Check sheet for the modelled part. Datum: model origin and axes. Units: mm. Face numbers are marked on the shaded views. A direction names the side the tool comes from. Round coordinates to 2 decimals unless told otherwise and drop trailing zeros. Write each loop counter-clockwise with the first axis right and the second up, starting at its lowest first coordinate (ties: lowest second). Pieces come first, ordered by that corner, then holes. Notation, with made-up numbers: (-21, -18.75) -> (18, -18.75) arc R21 cw to (18, 11.25) -> close; hole circle Ø2 at (-10.75, 49). An arc over 180 degrees is marked (long way). One line per item, written item: value.
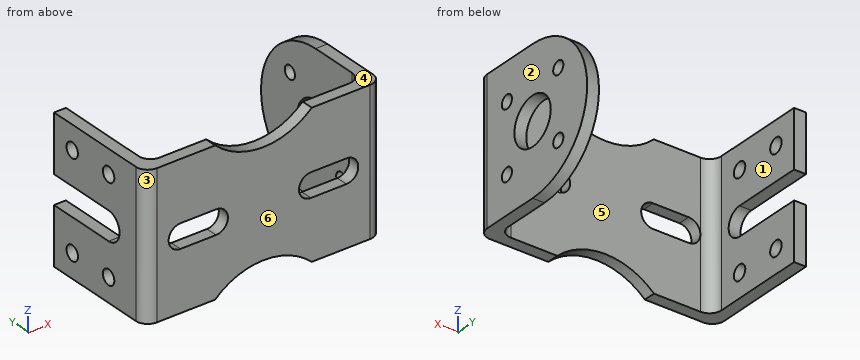
from build123d import *

# Parameters (mm, degrees)
SALIENTE_EXTRUIR1_DEPTH = 5
CROQUIS2_R              = 10.000000000000002
CROQUIS2_R_2            = 2.7999999999999976
CROQUIS2_R_3            = 2.800000000000002
SALIENTE_EXTRUIR2_DEPTH = 5
CROQUIS3_R              = 3.149999999999999
CROQUIS3_R_2            = 3.1499999999999972
SALIENTE_EXTRUIR3_DEPTH = 5
REDONDEO1_R             = 5
REDONDEO2_R             = 5
REDONDEO3_R             = 5
REDONDEO4_R             = 5


with BuildPart() as part:
    # Croquis1 → Saliente-Extruir1 (new body)
    with BuildSketch(Plane(origin=(0, 0, 0), x_dir=(1, 0, 0), z_dir=(0, 1, 0))):
        with BuildLine():
            Line((-46.42082429501085, 21.041214750542295), (-16.81690234938199, 21.041214750542295))
            ThreePointArc((-16.81690234938199, 21.041214750542295), (3.579175704989149, 13.041214750542295), (23.975253759360285, 21.041214750542295))
            Line((23.975253759360285, 21.041214750542295), (53.57917570498915, 21.041214750542295))
            Line((53.57917570498915, 21.041214750542295), (53.57917570498915, -38.9587852494577))
            Line((53.57917570498915, -38.9587852494577), (23.975253759360285, -38.9587852494577))
            ThreePointArc((23.975253759360285, -38.9587852494577), (3.579175704989149, -30.958785249457698), (-16.81690234938199, -38.9587852494577))
            Line((-16.81690234938199, -38.9587852494577), (-46.420824295010846, -38.9587852494577))
            Line((-46.420824295010846, -38.9587852494577), (-46.42082429501085, 21.041214750542295))
        make_face()
        with BuildLine():
            Line((-16.42082429501085, -3.958785249457704), (-31.42082429501085, -3.9587852494577107))
            ThreePointArc((-31.42082429501085, -3.9587852494577107), (-36.420824295010846, -8.958785249457705), (-31.42082429501085, -13.9587852494577))
            Line((-31.42082429501085, -13.9587852494577), (-16.42082429501085, -13.958785249457705))
            ThreePointArc((-16.42082429501085, -13.958785249457705), (-11.42082429501085, -8.958785249457705), (-16.42082429501085, -3.958785249457704))
        make_face(mode=Mode.SUBTRACT)
        with BuildLine():
            Line((23.579175704989144, -13.958785249457705), (38.57917570498914, -13.9587852494577))
            ThreePointArc((38.57917570498914, -13.9587852494577), (43.57917570498913, -8.958785249457705), (38.57917570498914, -3.9587852494577107))
            Line((38.57917570498914, -3.9587852494577107), (23.579175704989144, -3.958785249457704))
            ThreePointArc((23.579175704989144, -3.958785249457704), (18.579175704989144, -8.958785249457705), (23.579175704989144, -13.958785249457705))
        make_face(mode=Mode.SUBTRACT)
    extrude(amount=SALIENTE_EXTRUIR1_DEPTH)

    # Croquis2 → Saliente-Extruir2 (add)
    with BuildSketch(Plane(origin=(53.57917570498915, 0, 0), x_dir=(0, 0, -1), z_dir=(1, 0, 0))):
        with BuildLine():
            Line((-38.9587852494577, 0), (21.0412147505423, 0))
            Line((21.0412147505423, 0), (21.0412147505423, 30))
            ThreePointArc((21.0412147505423, 30), (-8.9587852494577, 60), (-38.9587852494577, 30))
            Line((-38.9587852494577, 30), (-38.9587852494577, 0))
        make_face()
        with Locations((-8.958785249457701, 30)):
            Circle(CROQUIS2_R, mode=Mode.SUBTRACT)
        with Locations((-23.10092087318865, 44.14213562373096)):
            Circle(CROQUIS2_R_2, mode=Mode.SUBTRACT)
        with Locations((-23.100920873188652, 15.85786437626905)):
            Circle(CROQUIS2_R_3, mode=Mode.SUBTRACT)
        with Locations(Location((5.183350374273251, 15.85786437626905, 0), (0, 0, 180))):
            Circle(CROQUIS2_R_3, mode=Mode.SUBTRACT)
        with Locations(Location((5.183350374273248, 44.14213562373096, 0), (0, 0, 180))):
            Circle(CROQUIS2_R_2, mode=Mode.SUBTRACT)
    extrude(amount=-SALIENTE_EXTRUIR2_DEPTH)

    # Croquis3 → Saliente-Extruir3 (add)
    with BuildSketch(Plane.ZY.offset(46.42082429501085)):
        with BuildLine():
            Line((-21.041214750542302, 0), (38.9587852494577, 0))
            Line((38.9587852494577, 0), (38.9587852494577, 50))
            Line((38.9587852494577, 50), (14.958785249457705, 50))
            Line((14.958785249457705, 50), (14.958785249457707, 20.000000000000004))
            ThreePointArc((14.958785249457707, 20.000000000000004), (8.958785249457703, 14.000000000000004), (2.958785249457704, 20.000000000000004))
            Line((2.958785249457704, 20.000000000000004), (2.9587852494577036, 50))
            Line((2.9587852494577036, 50), (-21.041214750542302, 50))
            Line((-21.041214750542302, 50), (-21.041214750542302, 0))
        make_face()
        with Locations((-11.041214750542295, 19.999999999999996)):
            Circle(CROQUIS3_R, mode=Mode.SUBTRACT)
        with Locations((-11.041214750542295, 39.99999999999999)):
            Circle(CROQUIS3_R, mode=Mode.SUBTRACT)
        with Locations(Location((28.958785249457705, 20.000000000000004, 0), (0, 0, 180))):
            Circle(CROQUIS3_R, mode=Mode.SUBTRACT)
        with Locations(Location((28.958785249457698, 40.00000000000001, 0), (0, 0, 180))):
            Circle(CROQUIS3_R_2, mode=Mode.SUBTRACT)
    extrude(amount=-SALIENTE_EXTRUIR3_DEPTH)

    # Redondeo1
    redondeo1_edges = [part.edges().sort_by_distance(p)[0] for p in [
        (-41.42082429501085, 5, 8.9587852494577),
    ]]
    fillet(redondeo1_edges, radius=REDONDEO1_R)

    # Redondeo2
    redondeo2_edges = [part.edges().sort_by_distance(p)[0] for p in [
        (48.57917570498915, 5, 8.958785249457703),
    ]]
    fillet(redondeo2_edges, radius=REDONDEO2_R)

    # Redondeo3
    redondeo3_edges = [part.edges().sort_by_distance(p)[0] for p in [
        (53.57917570498915, 0, 8.958785249457701),
    ]]
    fillet(redondeo3_edges, radius=REDONDEO3_R)

    # Redondeo4
    redondeo4_edges = [part.edges().sort_by_distance(p)[0] for p in [
        (-46.420824295010846, 0, 8.958785249457701),
    ]]
    fillet(redondeo4_edges, radius=REDONDEO4_R)


solid = part.part
Item 1: Tool access check on the marked faces 5 and 6. Record the directions out of +Z, -Z, +X, -X, +Y, -Y that give a thin tool (end or side, any length) a straight path to the whole face; none if there is none.
Result set:
face 5: +Z, -Z, +Y
face 6: +Z, -Z, +X, -X, -Y
Item 2: Sectioned sample at A-A (x = 37.5). Enter the section's corners in (y, z).
Result set:
outline: (0, -21.04) -> (5, -21.04) -> (5, 3.96) -> (0, 3.96) -> close; (0, 13.96) -> (5, 13.96) -> (5, 38.96) -> (0, 38.96) -> close
Item 3: Release check for a two-part mould opening along X. For the marked faces 1, 2, 3 and 4 record: pulls with the +X half, pulls with the -X half, needs draft (parallel to the pull), parting line crosses it, or undercut.
Result set:
face 1: undercut
face 2: pulls with the +X half
face 3: pulls with the -X half
face 4: needs draft
Item 4: Sectioned sample at B-B (z = -16.5). Enter the section's corners in (x, y), then the cut area to 3 significant figures.
Result set:
outline: (-46.42, 5) arc R5 ccw to (-41.42, 0) -> (-10.41, 0) -> (-10.41, 5) -> (-36.42, 5) arc R5 cw to (-41.42, 10) -> (-41.42, 50) -> (-46.42, 50) -> close; (17.56, 0) -> (48.58, 0) arc R5 ccw to (53.58, 5) -> (53.58, 45.87) -> (48.58, 45.87) -> (48.58, 10) arc R5 cw to (43.58, 5) -> (17.56, 5) -> close
area: 790 mm^2
Item 5: Sectioned sample at C-C (z = 27). Enter the section's corners in (x, y).
Result set:
outline: (-46.42, 5) arc R5 ccw to (-41.42, 0) -> (48.58, 0) arc R5 ccw to (53.58, 5) -> (53.58, 53.97) -> (48.58, 53.97) -> (48.58, 10) arc R5 cw to (43.58, 5) -> (-36.42, 5) arc R5 cw to (-41.42, 10) -> (-41.42, 17.53) -> (-46.42, 17.53) -> close; (-46.42, 22.47) -> (-41.42, 22.47) -> (-41.42, 37.53) -> (-46.42, 37.53) -> close; (-46.42, 42.47) -> (-41.42, 42.47) -> (-41.42, 50) -> (-46.42, 50) -> close
Item 6: Sectioned sample at D-D (x = 9.5). Enter the section's corners in (y, z).
Result set:
outline: (0, -13.63) -> (5, -13.63) -> (5, 31.55) -> (0, 31.55) -> close
Item 7: Depth check by flat-ended pin: pin 1 (7 mm diameter, centred on y = 40, z = 28.96, fed in from -X); pin 2 (18 mm diameter, centred on x = 23, z = 16, fed in from +Y); pin 3 (1.5 mm diameter, centred on x = -44, z = -3, fed in from +Y); pin 4 (4.5 mm diameter, centred on y = 44.14, z = -5.18, fed in from +X). Enter the tip coordinate at first touch or a pass-through.
Result set:
pin 1: x = -46.42
pin 2: y = 5
pin 3: y = 50
pin 4: x = -41.42
Item 8: Material ranges on line 1 along X through (y, z) = (38, 21); line 2 along X through (y, z) = (51, 13.5); line 3 along Y through (x, z) = (-14, -6.5), recorded low to high.
Result set:
line 1: -46.42 to -41.42, 48.58 to 53.58
line 2: 48.58 to 53.58
line 3: 0 to 5
